```python
from build123d import *

# Parameters (mm, degrees)
F1_DEPTH     = 156
F2_W         = 150
F2_H         = 70
F3_DEPTH     = 16
F4_T1_DEPTH  = 152
F4_T3_DEPTH  = 51
F4_T5_DEPTH  = 166
F4_T7_DEPTH  = 78
F4_T9_DEPTH  = 71
F4_T11_DEPTH = 79
F4_T13_DEPTH = 15
F4_S17_W     = 2
F4_S17_H     = 2
F4_T18_DEPTH = 2
F4_S23_W     = 2
F4_S23_H     = 2
F4_T24_DEPTH = 2
F4_S29_W     = 2
F4_S29_H     = 2
F4_T30_DEPTH = 2
F4_S35_W     = 2
F4_S35_H     = 2
F4_T36_DEPTH = 2
F4_S41_W     = 2
F4_S41_H     = 2
F4_T42_DEPTH = 2
F4_S47_W     = 2
F4_S47_H     = 2
F4_T48_DEPTH = 2
F4_T55_DEPTH = 83
F4_T59_DEPTH = 76
F4_T66_DEPTH = 83
F4_T70_DEPTH = 76


# Not quite as in the source:
# - a fillet or chamfer that OpenCascade refuses, or shapes differently, is made with other operations: its cross-section is extruded or revolved along the edge and cut away or added


with BuildPart() as f1:
    # F0 (on Right) → F1 (new body)
    with BuildSketch(Plane.YZ):
        Polygon((3, -99), (3, -3), (0, -3), (0, -80), (-73, -80), (-73, -99), align=None)
        Polygon((0, -3), (3, -3), (45, -3), (45, 0), (0, 0), align=None)
        Polygon((45, 0), (45, -3), (45, -33), (48, -33), (48, 0), align=None)
    extrude(amount=F1_DEPTH)

    # F2 (on face) → F3 (cut)
    with BuildSketch(Plane.XY.offset(-80)):
        with Locations((78, -35)):
            Rectangle(F2_W, F2_H)
    extrude(amount=-F3_DEPTH, mode=Mode.SUBTRACT)

    # F4: fillet of radius 2 on 16 edges, made by hand

    # F4_s2 → F4_t1 (cut)
    with BuildSketch(Plane.YZ.offset(2)):
        with BuildLine():
            ThreePointArc((2, 0), (0.5857864376, -0.5857864376), (0, -2))
            Line((0, -2), (0, 0))
            Line((0, 0), (2, 0))
        make_face()
        with BuildLine():
            ThreePointArc((-73, -82), (-72.4142135624, -80.5857864376), (-71, -80))
            Line((-71, -80), (-73, -80))
            Line((-73, -80), (-73, -82))
        make_face()
        with BuildLine():
            ThreePointArc((-71, -99), (-72.4142135624, -98.4142135624), (-73, -97))
            Line((-73, -97), (-73, -99))
            Line((-73, -99), (-71, -99))
        make_face()
    extrude(amount=F4_T1_DEPTH, mode=Mode.SUBTRACT)

    # F4_s4 → F4_t3 (cut)
    with BuildSketch(Plane.XZ.offset(-53)):
        with BuildLine():
            ThreePointArc((156, -2), (155.4142135624, -0.5857864376), (154, 0))
            Line((154, 0), (156, 0))
            Line((156, 0), (156, -2))
        make_face()
        with BuildLine():
            ThreePointArc((0, -2), (0.5857864376, -0.5857864376), (2, 0))
            Line((2, 0), (0, 0))
            Line((0, 0), (0, -2))
        make_face()
    extrude(amount=F4_T3_DEPTH, mode=Mode.SUBTRACT)

    # F4_s6 → F4_t5 (cut)
    with BuildSketch(Plane.YZ.offset(-5)):
        with BuildLine():
            ThreePointArc((48, -2), (47.4142135624, -0.5857864376), (46, 0))
            Line((46, 0), (48, 0))
            Line((48, 0), (48, -2))
        make_face()
        with BuildLine():
            ThreePointArc((46, -33), (47.4142135624, -32.4142135624), (48, -31))
            Line((48, -31), (48, -33))
            Line((48, -33), (46, -33))
        make_face()
        with BuildLine():
            ThreePointArc((45, -31), (45.5857864376, -32.4142135624), (47, -33))
            Line((47, -33), (45, -33))
            Line((45, -33), (45, -31))
        make_face()
    extrude(amount=F4_T5_DEPTH, mode=Mode.SUBTRACT)

    # F4_s8 → F4_t7 (cut)
    with BuildSketch(Plane.XY.offset(-80)):
        with BuildLine():
            ThreePointArc((156, 2), (155.4142135624, 0.5857864376), (154, 0))
            Line((154, 0), (156, 0))
            Line((156, 0), (156, 2))
        make_face()
        with BuildLine():
            ThreePointArc((0, 2), (0.5857864376, 0.5857864376), (2, 0))
            Line((2, 0), (0, 0))
            Line((0, 0), (0, 2))
        make_face()
    extrude(amount=F4_T7_DEPTH, mode=Mode.SUBTRACT)

    # F4_s10 → F4_t9 (cut)
    with BuildSketch(Plane.XZ):
        with BuildLine():
            ThreePointArc((156, -82), (155.4142135624, -80.5857864376), (154, -80))
            Line((154, -80), (156, -80))
            Line((156, -80), (156, -82))
        make_face()
        with BuildLine():
            ThreePointArc((0, -82), (0.5857864376, -80.5857864376), (2, -80))
            Line((2, -80), (0, -80))
            Line((0, -80), (0, -82))
        make_face()
    extrude(amount=F4_T9_DEPTH, mode=Mode.SUBTRACT)

    # F4_s12 → F4_t11 (cut)
    with BuildSketch(Plane.XZ.offset(-8)):
        with BuildLine():
            ThreePointArc((154, -99), (155.4142135624, -98.4142135624), (156, -97))
            Line((156, -97), (156, -99))
            Line((156, -99), (154, -99))
        make_face()
        with BuildLine():
            ThreePointArc((2, -99), (0.5857864376, -98.4142135624), (0, -97))
            Line((0, -97), (0, -99))
            Line((0, -99), (2, -99))
        make_face()
    extrude(amount=F4_T11_DEPTH, mode=Mode.SUBTRACT)

    # F4_s14 → F4_t13 (cut)
    with BuildSketch(Plane.XY.offset(-97)):
        with BuildLine():
            ThreePointArc((0, -71), (0.5857864376, -72.4142135624), (2, -73))
            Line((2, -73), (0, -73))
            Line((0, -73), (0, -71))
        make_face()
        with BuildLine():
            ThreePointArc((156, -71), (155.4142135624, -72.4142135624), (154, -73))
            Line((154, -73), (156, -73))
            Line((156, -73), (156, -71))
        make_face()
    extrude(amount=F4_T13_DEPTH, mode=Mode.SUBTRACT)


with BuildPart() as f4_tool16:
    # F4_s17 → F4_t18 (new body)
    with BuildSketch(Plane.XY.offset(-2)):
        with Locations((1, 1)):
            Rectangle(F4_S17_W, F4_S17_H)
    extrude(amount=F4_T18_DEPTH)

    # F4_s19 → F4_t20 (revolve, cut)
    with BuildSketch(Plane(origin=(2, 2, -2), x_dir=(0.7071067812, 0.7071067812, 0), z_dir=(0.7071067812, -0.7071067812, 0))):
        with BuildLine():
            ThreePointArc((0, -2), (2, 0), (0, 2))
            Line((0, 2), (0, -2))
        make_face()
    revolve(axis=Axis((2, 2, -2), (0, 0, 1)), mode=Mode.SUBTRACT)


with BuildPart() as f1_1:
    add(f1.part)

    # F4_t15: cut F4_tool16
    add(f4_tool16.part, mode=Mode.SUBTRACT)


with BuildPart() as f4_tool22:
    # F4_s23 → F4_t24 (new body)
    with BuildSketch(Plane.XY.offset(-2)):
        with Locations((155, 1)):
            Rectangle(F4_S23_W, F4_S23_H)
    extrude(amount=F4_T24_DEPTH)

    # F4_s25 → F4_t26 (revolve, cut)
    with BuildSketch(Plane(origin=(154, 2, -2), x_dir=(-0.7071067812, 0.7071067812, 0), z_dir=(0.7071067812, 0.7071067812, 0))):
        with BuildLine():
            ThreePointArc((0, -2), (2, 0), (0, 2))
            Line((0, 2), (0, -2))
        make_face()
    revolve(axis=Axis((154, 2, -2), (0, 0, 1)), mode=Mode.SUBTRACT)


with BuildPart() as f1_2:
    add(f1_1.part)

    # F4_t21: cut F4_tool22
    add(f4_tool22.part, mode=Mode.SUBTRACT)


with BuildPart() as f4_tool28:
    # F4_s29 → F4_t30 (new body)
    with BuildSketch(Plane.XY.offset(-82)):
        with Locations((155, -72)):
            Rectangle(F4_S29_W, F4_S29_H)
    extrude(amount=F4_T30_DEPTH)

    # F4_s31 → F4_t32 (revolve, cut)
    with BuildSketch(Plane(origin=(154, -71, -82), x_dir=(-0.7071067812, 0.7071067812, 0), z_dir=(0.7071067812, 0.7071067812, 0))):
        with BuildLine():
            ThreePointArc((0, -2), (2, 0), (0, 2))
            Line((0, 2), (0, -2))
        make_face()
    revolve(axis=Axis((154, -71, -82), (0, 0, 1)), mode=Mode.SUBTRACT)


with BuildPart() as f1_3:
    add(f1_2.part)

    # F4_t27: cut F4_tool28
    add(f4_tool28.part, mode=Mode.SUBTRACT)


with BuildPart() as f4_tool34:
    # F4_s35 → F4_t36 (new body)
    with BuildSketch(Plane.YZ.offset(2)):
        with Locations((-72, -81)):
            Rectangle(F4_S35_W, F4_S35_H)
    extrude(amount=-F4_T36_DEPTH)

    # F4_s37 → F4_t38 (revolve, cut)
    with BuildSketch(Plane(origin=(2, -71, -82), x_dir=(0, 0.7071067812, -0.7071067812), z_dir=(0, 0.7071067812, 0.7071067812))):
        with BuildLine():
            ThreePointArc((0, -2), (2, 0), (0, 2))
            Line((0, 2), (0, -2))
        make_face()
    revolve(axis=Axis((2, -71, -82), (-1, 0, 0)), mode=Mode.SUBTRACT)


with BuildPart() as f1_4:
    add(f1_3.part)

    # F4_t33: cut F4_tool34
    add(f4_tool34.part, mode=Mode.SUBTRACT)


with BuildPart() as f4_tool40:
    # F4_s41 → F4_t42 (new body)
    with BuildSketch(Plane.XY.offset(-97)):
        with Locations((1, -72)):
            Rectangle(F4_S41_W, F4_S41_H)
    extrude(amount=-F4_T42_DEPTH)

    # F4_s43 → F4_t44 (revolve, cut)
    with BuildSketch(Plane(origin=(2, -71, -97), x_dir=(0.7071067812, 0.7071067812, 0), z_dir=(-0.7071067812, 0.7071067812, 0))):
        with BuildLine():
            ThreePointArc((0, -2), (2, 0), (0, 2))
            Line((0, 2), (0, -2))
        make_face()
    revolve(axis=Axis((2, -71, -97), (0, 0, -1)), mode=Mode.SUBTRACT)


with BuildPart() as f1_5:
    add(f1_4.part)

    # F4_t39: cut F4_tool40
    add(f4_tool40.part, mode=Mode.SUBTRACT)


with BuildPart() as f4_tool46:
    # F4_s47 → F4_t48 (new body)
    with BuildSketch(Plane.XY.offset(-97)):
        with Locations((155, -72)):
            Rectangle(F4_S47_W, F4_S47_H)
    extrude(amount=-F4_T48_DEPTH)

    # F4_s49 → F4_t50 (revolve, cut)
    with BuildSketch(Plane(origin=(154, -71, -97), x_dir=(-0.7071067812, 0.7071067812, 0), z_dir=(-0.7071067812, -0.7071067812, 0))):
        with BuildLine():
            ThreePointArc((0, -2), (2, 0), (0, 2))
            Line((0, 2), (0, -2))
        make_face()
    revolve(axis=Axis((154, -71, -97), (0, 0, -1)), mode=Mode.SUBTRACT)


with BuildPart() as f1_6:
    add(f1_5.part)

    # F4_t45: cut F4_tool46
    add(f4_tool46.part, mode=Mode.SUBTRACT)


with BuildPart() as f4_tool53:
    # F4_s54 → F4_t55 (new body)
    with BuildSketch(Plane.XY.offset(-2)):
        with BuildLine():
            ThreePointArc((156, 2), (155.4142135624, 0.5857864376), (154, 0))
            Line((154, 0), (156, 0))
            Line((156, 0), (156, 2))
        make_face()
    extrude(amount=-F4_T55_DEPTH)

    split(bisect_by=Plane.XY.offset(-80), keep=Keep.BOTTOM)


with BuildPart() as f4_tool57:
    # F4_s58 → F4_t59 (new body)
    with BuildSketch(Plane.XZ.offset(-5)):
        with BuildLine():
            ThreePointArc((156, -82), (155.4142135624, -80.5857864376), (154, -80))
            Line((154, -80), (156, -80))
            Line((156, -80), (156, -82))
        make_face()
    extrude(amount=F4_T59_DEPTH)

    split(bisect_by=Plane.XZ, keep=Keep.BOTTOM)


with BuildPart() as f4_tool53_1:
    add(f4_tool53.part)

    # F4_t61: intersect F4_tool57
    add(f4_tool57.part, mode=Mode.INTERSECT)


with BuildPart() as f1_7:
    add(f1_6.part)

    # F4_t51: cut F4_tool53
    add(f4_tool53_1.part, mode=Mode.SUBTRACT)


with BuildPart() as f4_tool64:
    # F4_s65 → F4_t66 (new body)
    with BuildSketch(Plane.XY.offset(-2)):
        with BuildLine():
            ThreePointArc((0, 2), (0.5857864376, 0.5857864376), (2, 0))
            Line((2, 0), (0, 0))
            Line((0, 0), (0, 2))
        make_face()
    extrude(amount=-F4_T66_DEPTH)

    split(bisect_by=Plane.XY.offset(-80), keep=Keep.BOTTOM)


with BuildPart() as f4_tool68:
    # F4_s69 → F4_t70 (new body)
    with BuildSketch(Plane.XZ.offset(-5)):
        with BuildLine():
            ThreePointArc((0, -82), (0.5857864376, -80.5857864376), (2, -80))
            Line((2, -80), (0, -80))
            Line((0, -80), (0, -82))
        make_face()
    extrude(amount=F4_T70_DEPTH)

    split(bisect_by=Plane.XZ, keep=Keep.BOTTOM)


with BuildPart() as f4_tool64_1:
    add(f4_tool64.part)

    # F4_t72: intersect F4_tool68
    add(f4_tool68.part, mode=Mode.INTERSECT)


with BuildPart() as f1_8:
    add(f1_7.part)

    # F4_t62: cut F4_tool64
    add(f4_tool64_1.part, mode=Mode.SUBTRACT)


solid = f1_8.part
```
Source: CAD feature listing. Evaluate the final solid. Frame: model axes, mm. A direction names the side the tool comes from. Coordinates: 2 decimals unless noted, no trailing zeros. Loops run counter-clockwise (first coordinate to the right, second up) from the corner with the lowest first, then second, coordinate; pieces in that order, holes last. Notation, with made-up numbers: (18.25, -27.5) - (77.25, -27.5) arc R28 ccw to (77.25, 7.5) - close; hole circle Ø5 at (-6, 18). An arc over 180 degrees is marked (long way). Answer as CSV lines item,"result".
1. Reachability of faces 4 (the flat face through (77, 45, -17)), 5 (the flat face through (0, -25, -84)), 6 (the flat face through (77, -35, -96)) from +Z, -Z, +X, -X, +Y, -Y: full face, straight path, thin tool, end or side. Return the list, or none.
Established:
face 4,"-Z, +X, -X"
face 5,"+Z, -Z, -X, +Y, -Y"
face 6,"+Z"
2. Contact query for flat-ended pins moving along their axis: pin 1 (6 mm diameter, centred on x = 101, z = -52.5, fed in from -Y); pin 2 (17.5 mm diameter, centred on x = 86, z = -88, fed in from +Y). Output: stop coordinate, or through.
Established:
pin 1,"stops at y = 0"
pin 2,"stops at y = 3"
3. Ray query, line 1 (X direction, y = -52.5, z = -93); line 2 (Y direction, x = 50, z = -84); line 3 (Y direction, x = 56, z = -15). Return the intervals inside material, ascending.
Established:
line 1,"x = 0 to 3, 153 to 156"
line 2,"y = -73 to -70, 0 to 3"
line 3,"y = 0 to 3, 45 to 48"
4. Section A-A (z = -27). Return loops of the section in (x, y).
Established:
outline,"(0, 2) arc R2 ccw to (2, 0) - (154, 0) arc R2 ccw to (156, 2) - (156, 3) - (0, 3) - close; (0, 45) - (156, 45) - (156, 48) - (0, 48) - close"
5. Mould query, pull axis X, two halves, no side actions, for faces 1 (the flat face through (77, 48, -17)), 2 (the flat face through (156, -25, -84)), 3 (the flat face through (77, -70, -88)). Classes: released by +X, released by -X, zero draft, split by the parting line, or undercut.
Established:
face 1,"zero draft"
face 2,"released by +X"
face 3,"undercut"
6. Section C-C (x = 51.5). Return loops of the section in (y, z).
Established:
outline,"(-73, -97) arc R2 ccw to (-71, -99) - (3, -99) - (3, -3) - (45, -3) - (45, -31) arc R2 ccw to (46.5, -32.94) arc R2 ccw to (48, -31) - (48, -2) arc R2 ccw to (46, 0) - (2, 0) arc R2 ccw to (0, -2) - (0, -96) - (-70, -96) - (-70, -80) - (-71, -80) arc R2 ccw to (-73, -82) - close"
7. Section D-D (y = 23). Return loops of the section in (x, z), then the cut area to 3 significant figures.
Established:
outline,"(0, -3) - (156, -3) - (156, -2) arc R2 ccw to (154, 0) - (2, 0) arc R2 ccw to (0, -2) - close"
area,"466 mm2"
8. Section B-B (y = -35.5). Return loops of the section in (x, z).
Established:
outline,"(0, -97) arc R2 ccw to (2, -99) - (154, -99) arc R2 ccw to (156, -97) - (156, -82) arc R2 ccw to (154, -80) - (153, -80) - (153, -96) - (3, -96) - (3, -80) - (2, -80) arc R2 ccw to (0, -82) - close"
